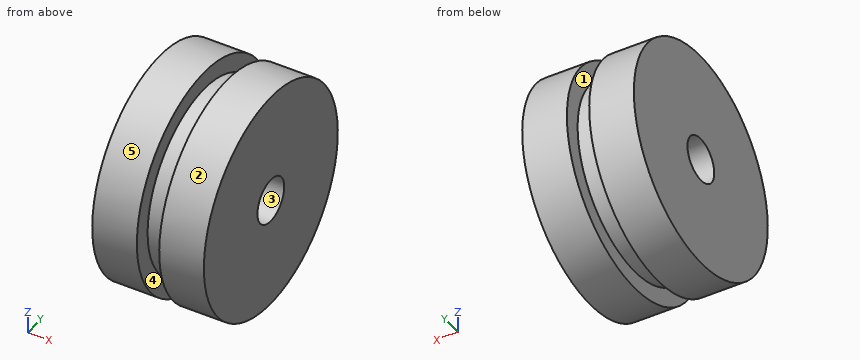
from build123d import *

# Parameters (mm, degrees)
F3_D = 2


with BuildPart() as f1:
    # F0 (on Front) → F1 (revolve)
    with BuildSketch(Plane.XZ):
        Polygon((-2.5, 5), (-2.5, 0), (2.5, 0), (2.5, 5), (0.5, 5), (0.5, 4.2), (-0.5, 4.2), (-0.5, 5), align=None)
    revolve(axis=Axis((0.0154641815, 0, 0), (1, 0, 0)))

    # F3 (through all)
    with Locations(Plane(origin=(-2.5, 0, 0), x_dir=(0, -1, 0), z_dir=(-1, 0, 0))):
        with Locations((0, 0)):
            Hole(F3_D / 2)


solid = f1.part
Source: CAD feature listing. Evaluate the final solid. Frame: model axes, mm. Face numbers are marked on the shaded views. A direction names the side the tool comes from. Round coordinates to 2 decimals unless told otherwise and drop trailing zeros. Loops run counter-clockwise (first coordinate to the right, second up) from the corner with the lowest first, then second, coordinate; pieces in that order, holes last. Notation, with made-up numbers: M -39,41.5 L 5,41.5 A29 cw 5,79.5 Z; hole C 68,82.25 d1. An arc over 180 degrees is marked long. Return JSON: item names as keys, results as strings. Group by question number.
1. Section query A-A on z = 0. Output: boundary loops of the cut face in (x, y).
2. Pin query (flat end, axial travel): pin 1 (2.5 mm diameter, centred on y = 0, z = 0, fed in from +X); pin 2 (2 mm diameter, centred on x = 0, y = 1.5, fed in from -Z); pin 3 (3 mm diameter, centred on x = -2, z = 2, fed in from +Y). Return the tip coordinate at first contact, or that it passes through.
3. Mould query, pull axis Y, two halves, no side actions, for the marked faces 1, 2 and 3. Classes: released by +Y, released by -Y, zero draft, split by the parting line, or undercut.
4. Material intervals for line 1 along Z through (x, y) = (0.2, 0); line 2 along X through (y, z) = (-4.25, -2.25); line 3 along Z through (x, y) = (1.2, 0), sorted ascending. Write a range as from..to.
5. Section query B-B on x = 1.35. Output: boundary loops of the cut face in (y, z).
6. Section query C-C on y = 4. Output: boundary loops of the cut face in (x, z).
7. Reachability of the marked faces 4 and 5 from +Z, -Z, +X, -X, +Y, -Y: full face, straight path, thin tool, end or side. Return the list, or none.
Checks:
{
 "1": {"outline": "M -2.5,-5 L -0.5,-5 L -0.5,-4.2 L 0.5,-4.2 L 0.5,-5 L 2.5,-5 L 2.5,-1 L -2.5,-1 Z; M -2.5,1 L 2.5,1 L 2.5,5 L 0.5,5 L 0.5,4.2 L -0.5,4.2 L -0.5,5 L -2.5,5 Z"},
 "2": {"pin 1": "stops at x = 2.5", "pin 2": "stops at z = -4.96", "pin 3": "stops at y = 4.97"},
 "3": {"face 1": "zero draft", "face 2": "split by the parting line", "face 3": "undercut"},
 "4": {"line 1": "z = -4.2..-1, 1..4.2", "line 2": "x = -2.5..-0.5, 0.5..2.5", "line 3": "z = -5..-1, 1..5"},
 "5": {"outline": "C 0,0 d10; hole C 0,0 d2"},
 "6": {"outline": "M -2.5,-3 L -0.5,-3 L -0.5,-1.28 L 0.5,-1.28 L 0.5,-3 L 2.5,-3 L 2.5,3 L 0.5,3 L 0.5,1.28 L -0.5,1.28 L -0.5,3 L -2.5,3 Z"},
 "7": {"face 4": "none", "face 5": "+X, -X"}
}
